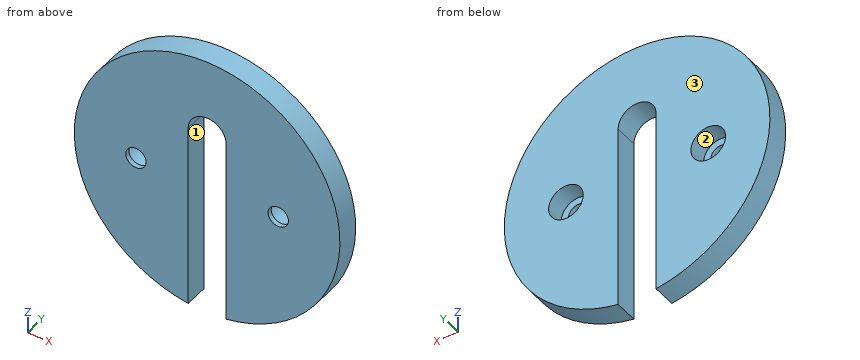
```python
from build123d import *

# Parameters (mm, degrees)
F0_R     = 28
F1_DEPTH = 5
F3_DEPTH = 35
F4_R     = 2.15
F5_DEPTH = 25
F6_R     = 3.65
F7_DEPTH = 4


with BuildPart() as f1:
    # F0 (on Front) → F1 (new body)
    with BuildSketch(Plane.XZ):
        Circle(F0_R)
    extrude(amount=F1_DEPTH)

    # F2 (on face) → F3 (cut)
    with BuildSketch(Plane(origin=(0, 0, 0), x_dir=(-1, 0, 0), z_dir=(0, 1, 0))):
        with BuildLine():
            ThreePointArc((4, 11.5), (0, 15.5), (-4, 11.5))
            Line((-4, 11.5), (-4, -27.712813))
            ThreePointArc((-4, -27.712813), (0, -28), (4, -27.712813))
            Line((4, -27.712813), (4, 11.5))
        make_face()
    extrude(amount=-F3_DEPTH, mode=Mode.SUBTRACT)

    # F4 (on face) → F5 (cut)
    with BuildSketch(Plane(origin=(0, 0, 0), x_dir=(-1, 0, 0), z_dir=(0, 1, 0))):
        with Locations((-15, 0)):
            Circle(F4_R)
        with Locations((15, 0)):
            Circle(F4_R)
    extrude(amount=-F5_DEPTH, mode=Mode.SUBTRACT)

    # F6 (on face) → F7 (cut)
    with BuildSketch(Plane(origin=(0, 0, 0), x_dir=(-1, 0, 0), z_dir=(0, 1, 0))):
        with Locations((-15, 0)):
            Circle(F6_R)
        with Locations((15, 0)):
            Circle(F6_R)
    extrude(amount=-F7_DEPTH, mode=Mode.SUBTRACT)


solid = f1.part
```
Model file for the job. Use its own axes, mm. Face numbers are marked on the shaded views. A direction names the side the tool comes from. Round coordinates to 2 decimals unless told otherwise and drop trailing zeros. Loops run counter-clockwise (first coordinate to the right, second up) from the corner with the lowest first, then second, coordinate; pieces in that order, holes last. Notation, with made-up numbers: M 87,-25 L 115,-25 A27 cw 115,9 Z; hole C -17,-36 d6. An arc over 180 degrees is marked long. Put each result on its own line as item: value. Start each with the question number.
Item 1: Cut at C-C (y = -3.2). List the corners of the cut face in (x, z).
Item 2: Cut at D-D (z = 9). List the corners of the cut face in (x, y).
Item 3: 3-axis set-ups, long thin cutter, end or side, ignore diameter. For the marked faces 1, 2 and 3: which of +Z, -Z, +X, -X, +Y, -Y reach the whole face in a straight line?
Item 4: Cut at B-B (x = 15). List the corners of the cut face in (y, z).
Item 5: Cut at A-A (z = 0). List the corners of the cut face in (x, y), then the cut area to 3 significant figures.
Item 6: Drill centre lines: line 1 along Z through (x, y) = (17, -3); line 2 along X through (y, z) = (-3.7, -19); line 3 along X through (y, z) = (-4.1, 6). Where is each one in solid material? Low to high.
Item 7: Drop flat-ended pins along their axis: P1, Ø5.5, axis at x = -15, z = 0, coming from the -Y side; P2, Ø1.5, axis at x = -6, y = -3, coming from the +Z side; P3, Ø2, axis at x = -16, z = -1.5, coming from the +Y side; P4, Ø1.5, axis at y = -2.5, z = -6.5, coming from the -X side. Give the stop position or say it passes through.
Answer block:
1. outline: M -4,-27.71 L -4,11.5 A4 cw 4,11.5 L 4,-27.71 A28 ccw long Z; hole C -15,0 d7.3; hole C 15,0 d7.3
2. outline: M -26.51,-5 L -4,-5 L -4,0 L -26.51,0 Z; M 4,-5 L 26.51,-5 L 26.51,0 L 4,0 Z
3. face 1: -Z, +Y, -Y
3. face 2: +Y
3. face 3: +Z, -Z, +X, -X, +Y
4. outline: M -5,-23.64 L 0,-23.64 L 0,-3.65 L -4,-3.65 L -4,-2.15 L -5,-2.15 Z; M -5,2.15 L -4,2.15 L -4,3.65 L 0,3.65 L 0,23.64 L -5,23.64 Z
5. outline: M -28,-5 L -17.15,-5 L -17.15,-4 L -18.65,-4 L -18.65,0 L -28,0 Z; M -12.85,-5 L -4,-5 L -4,0 L -11.35,0 L -11.35,-4 L -12.85,-4 Z; M 4,-5 L 12.85,-5 L 12.85,-4 L 11.35,-4 L 11.35,0 L 4,0 Z; M 17.15,-5 L 28,-5 L 28,0 L 18.65,0 L 18.65,-4 L 17.15,-4 Z
5. area: 173 mm2
6. line 1: -22.25 to -3.05, 3.05 to 22.25
6. line 2: -20.57 to -4, 4 to 20.57
6. line 3: -27.35 to -4, 4 to 27.35
7. P1: y = -5
7. P2: z = 27.5
7. P3: y = -4
7. P4: x = -27.4
